Geometry check sheet. Reference: the model listing, model coordinates, mm. Face numbers are marked on the shaded views. A direction names the side the tool comes from. Round coordinates to 2 decimals unless told otherwise and drop trailing zeros. Order: outer loops, then holes, each group sorted by start corner. A loop starts at its lowest first (then second) coordinate and runs counter-clockwise, first axis right, second up.
(1) Sectioned sample at D-D (x = 63.5). Record the boundary of the cut face in (y, z), plus the area to 3 significant figures.
(2) Sectioned sample at C-C (z = -11). Record the boundary of the cut face in (x, y), plus the area to 3 significant figures.
(3) Release check for a two-part mould opening along X. For the marked faces 4, 5 and 6 record: +X half, -X half, draft (parallel to the pull), parting line (faces both ways), or undercut.
(4) Go/stop test with flat-tipped pins: pin 1 (16.5 mm diameter, centred on x = 0, y = 0, fed in from -Z); pin 2 (3 mm diameter, centred on y = -20, z = -19, fed in from +X); pin 3 (11 mm diameter, centred on x = -5.5, y = -1, fed in from -Z); pin 4 (12 mm diameter, centred on x = 68.5, z = -9, fed in from -Y). Record where each tip stops, or that it passes through.
(5) Sectioned sample at A-A (z = -32). Record the boundary of the cut face in (x, y).
(6) Sectioned sample at B-B (y = -63). Record the boundary of the cut face in (x, z), plus the area to 3 significant figures.
(7) Material ranges on line 1 along X through (y, z) = (-29, -28); line 2 along X through (y, z) = (-14, -6); line 3 along Z through (x, y) = (9, -44), recorded low to high.
(8) Set-up check for the marked faces 1, 2 and 3: record each of +Z, -Z, +X, -X, +Y, -Y from which the full face is reachable in a straight line by a thin tool's end or side.
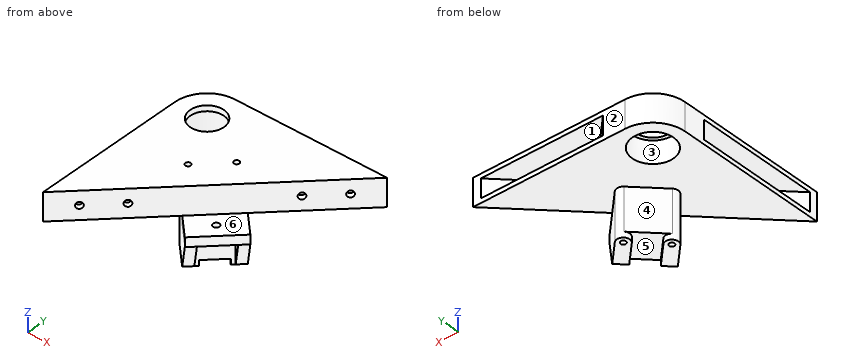
Autodesk Inventor part; units mm, degrees
ref_plane "YZ Plane" through (0, 0, 0) normal (1, 0, 0) x (0, 1, 0)
ref_plane "XZ Plane" through (0, 0, 0) normal (0, 1, 0) x (-1, 0, 0)
ref_plane "XY Plane" through (0, 0, 0) normal (0, 0, 1) x (1, 0, 0)
sketch "Sketch1" plane through (0, 0, 0) normal (0, 0, 1) x (1, 0, 0)
  circle A0 centre (0, 0) radius 4
  line L0 (-144.1925, -209.3609) -> (209.3609, 144.1925)
  circle A1 centre (0, 0) radius 11.15
  circle A2 centre (0, 0) radius 17.5
  line L1 (-17.5, 0) -> (-17.5, -82.6684)
  line L2 (0, 17.5) -> (82.6684, 17.5)
  point P0 (0, 0)
  dimension "d0" = 22.3
  dimension "d1" = 35
extrude "Extrusion1" add sketch "Sketch1" against normal blind 15 contours L1 A2 L2 L0 | A2
sketch "Sketch2" plane through (0, 0, 0) normal (0, 0, 1) x (1, 0, 0)
  arc A0 (0, 17.5) -> (-17.5, 0) centre (0, 0) ccw
  line L0 (-17.5, 0) -> (-17.5, -82.6684)
  line L1 (-17.5, -82.6684) -> (82.6684, 17.5)
  line L2 (82.6684, 17.5) -> (0, 17.5)
  circle A1 centre (0, 0) radius 11.15
  circle A2 centre (0, 0) radius 9.15
  dimension "d6" = 2
extrude "Extrusion2" add sketch "Sketch2" against normal blind 3 contours A1
ref_plane "Work Plane1" through (-19.6213, -80.5471, 0) normal (0.7071068, -0.7071068, 0) x (-0.7071068, -0.7071068, 0)
sketch "Sketch3" plane through (-19.6213, -80.5471, 0) normal (0.7071068, -0.7071068, 0) x (-0.7071068, -0.7071068, 0)
  line L0 (-141.6595, 0) -> (-83.2041, 0)
  line L1 (-141.6595, 0) -> (-141.6595, 15)
  line L2 (-83.2041, 15) -> (-141.6595, 15)
  line L3 (-83.2041, 0) -> (-83.2041, 15)
  line L4 (-58.4554, 0) -> (0, 0)
  line L5 (-58.4554, 0) -> (-58.4554, 15)
  line L6 (0, 15) -> (-58.4554, 15)
  line L7 (0, 0) -> (0, 15)
  line L8 (-83.2041, 0) -> (-58.4554, 0)
  line L9 (-50.8297, 15) -> (-90.8297, 15)
  line L10 (-141.6595, 0) -> (-141.6595, 15)
  line L11 (-141.6595, 12.6) -> (-91.6595, 12.6)
  line L12 (-91.6595, 12.6) -> (-91.6595, 2.4)
  line L13 (-91.6595, 2.4) -> (-141.6595, 2.4)
  line L14 (-141.6595, 2.4) -> (-141.6595, 12.6)
  line L15 (0, 0) -> (0, 15)
  line L16 (0, 2.4) -> (-50, 2.4)
  line L17 (-50, 2.4) -> (-50, 12.6)
  line L18 (-50, 12.6) -> (0, 12.6)
  line L19 (0, 12.6) -> (0, 2.4)
  point P0 (-70.8297, 0)
  point P1 (0, 12.6)
  dimension "d8" = 2.4
  dimension "d9" = 2.4
  dimension "d10" = 2.4
  dimension "d11" = 50
extrude "Extrusion3" cut sketch "Sketch3" against normal through all contours L1 L11 L12 L13 | L16 L17 L18 L7
sketch "Sketch4" plane through (-19.6213, -80.5471, 0) normal (-0.7071068, 0.7071068, 0) x (0, 0, 1)
  line L0 (-12.6, 138.6595) -> (-2.4, 138.6595)
  line L1 (-12.6, 91.6595) -> (-12.6, 138.6595)
  line L2 (-2.4, 91.6595) -> (-12.6, 91.6595)
  line L3 (-2.4, 138.6595) -> (-2.4, 91.6595)
  line L4 (-2.4, 3) -> (-12.6, 3)
  line L5 (-2.4, 50) -> (-2.4, 3)
  line L6 (-12.6, 50) -> (-2.4, 50)
  line L7 (-12.6, 3) -> (-12.6, 50)
  line L8 (-12.6, 50) -> (-2.4, 50)
  line L9 (-2.4, 91.6595) -> (-12.6, 91.6595)
  point P0 (0, 70.8297)
  point P1 (-7.5, 106.6595)
  point P2 (-7.5, 126.6595)
  point P3 (-7.5, 35)
  point P4 (-7.5, 15)
  point P5 (-7.5, 50)
  point P6 (-7.5, 91.6595)
  dimension "d14" = 15
  dimension "d15" = 15
  dimension "d16" = 20
  dimension "d17" = 20
hole "Hole1" at (55.7983, -5.1274, -7.5) at (69.9405, 9.0147, -7.5) at (5.1274, -55.7983, -7.5) at (-9.0147, -69.9405, -7.5) direction (0.7071068, -0.7071068, 0) diameter 3.6 end through all
sketch "Sketch5" plane through (0, 0, 0) normal (0, 0, 1) x (1, 0, 0)
  circle A0 centre (0, 0) radius 9.15
  arc A1 (0, 17.5) -> (-17.5, 0) centre (0, 0) ccw
  line L0 (-17.5, 0) -> (-17.5, -82.6684)
  line L1 (-17.5, -82.6684) -> (82.6684, 17.5)
  line L2 (82.6684, 17.5) -> (0, 17.5)
  line L3 (29, -14.8579) -> (14.8579, -29) construction
  dimension "d25" = 29
  dimension "d26" = 29
  dimension "d27" = 20
hole "Hole2" at (29, -14.8579, 0) at (14.8579, -29, 0) direction (0, 0, -1) diameter 2.9 end through all
sketch "Sketch6" plane through (0, 0, -15) normal (0, 0, -1) x (-1, 0, 0)
  circle A0 centre (-29, -14.8579) radius 1.45
  circle A1 centre (-14.8579, -29) radius 1.45
  arc A2 (17.5, 0) -> (0, 17.5) centre (0, 0) ccw
  line L0 (0, 17.5) -> (-82.6684, 17.5)
  line L1 (-82.6684, 17.5) -> (17.5, -82.6684)
  line L2 (17.5, -82.6684) -> (17.5, 0)
  circle A3 centre (0, 0) radius 11.15
  circle A4 centre (-14.8579, -29) radius 1.45
  circle A5 centre (-14.8579, -29) radius 3.5
  circle A6 centre (-29, -14.8579) radius 1.45
  circle A7 centre (-29, -14.8579) radius 3.5
  line L3 (-12.383, -31.4749) -> (-23.0382, -42.1301)
  line L4 (-17.3327, -26.5251) -> (-27.988, -37.1804)
  line L5 (-82.6684, 17.5) -> (17.5, -82.6684)
  line L6 (-31.4749, -12.383) -> (-42.1301, -23.0382)
  line L7 (-26.5251, -17.3327) -> (-37.1804, -27.988)
  point P0 (0, 0)
  dimension "d35" = 7
extrude "Extrusion4" add sketch "Sketch6" along normal blind 26 contours L1 L4 A5 L3 | L6 A7 L7 L1 | A5 | A7
sketch "Sketch7" plane through (0, 0, -15) normal (0, 0, -1) x (-1, 0, 0)
  line L0 (-26.5251, -17.3327) -> (-37.1804, -27.988)
  line L1 (-37.1804, -27.988) -> (-27.988, -37.1804)
  line L2 (-27.988, -37.1804) -> (-17.3327, -26.5251)
  arc A0 (-12.383, -31.4749) -> (-17.3327, -26.5251) centre (-14.8579, -29) ccw
  line L3 (-12.383, -31.4749) -> (-23.0382, -42.1301)
  line L4 (-23.0382, -42.1301) -> (17.5, -82.6684)
  line L5 (17.5, -82.6684) -> (17.5, 0)
  arc A1 (17.5, 0) -> (0, 17.5) centre (0, 0) ccw
  line L6 (0, 17.5) -> (-82.6684, 17.5)
  line L7 (-82.6684, 17.5) -> (-42.1301, -23.0382)
  line L8 (-42.1301, -23.0382) -> (-31.4749, -12.383)
  arc A2 (-26.5251, -17.3327) -> (-31.4749, -12.383) centre (-29, -14.8579) ccw
  circle A3 centre (0, 0) radius 11.15
  line L9 (-12.383, -26.5251) -> (-26.5251, -12.383)
  arc A4 (-26.5251, -17.3327) -> (-31.4749, -12.383) centre (-29, -14.8579) ccw
  point P0 (0, 0)
extrude "Extrusion5" add sketch "Sketch7" along normal blind 23 contours A2 L9 A0 L2 L1 L0
sketch "Sketch8" plane through (-17.5, -82.6684, 0) normal (0.7071068, -0.7071068, 0) x (-0.7071068, -0.7071068, 0)
  circle A0 centre (-35, 7.5) radius 1.8
  circle A1 centre (-106.6595, 7.5) radius 1.8
  circle A2 centre (-126.6595, 7.5) radius 1.8
  circle A3 centre (-15, 7.5) radius 1.8
  line L0 (0, 0) -> (-141.6595, 0)
  line L1 (0, 0) -> (0, 15)
  line L2 (-57.3297, 15) -> (0, 15)
  line L3 (-57.3297, 15) -> (-57.3297, 41)
  line L4 (-64.3297, 41) -> (-57.3297, 41)
  line L5 (-64.3297, 38) -> (-64.3297, 41)
  line L6 (-77.3297, 38) -> (-64.3297, 38)
  line L7 (-77.3297, 38) -> (-77.3297, 41)
  line L8 (-84.3297, 41) -> (-77.3297, 41)
  line L9 (-84.3297, 15) -> (-84.3297, 41)
  line L10 (-141.6595, 15) -> (-84.3297, 15)
  line L11 (-141.6595, 0) -> (-141.6595, 15)
  line L12 (-84.3297, 15) -> (-57.3297, 15)
  line L13 (-83.2041, 15) -> (-141.6595, 15)
  line L14 (-84.3297, 15) -> (-84.3297, 41)
  line L15 (-84.3297, 20) -> (-57.3297, 20)
  point P0 (-70.8297, 0)
  dimension "d40" = 5
extrude "Extrusion6" add sketch "Sketch8" along normal blind 15 contours L12 L9 L15 L3
sketch "Sketch9" plane through (31.4749, -12.383, -41) normal (0.7071068, 0.7071068, 0) x (-0.7071068, 0.7071068, 0)
  line L0 (-15.0688, 26) -> (0, 26)
  line L1 (-15.0688, 26) -> (-30.0688, 26)
  line L2 (-30.0688, 21) -> (-30.0688, 26)
  line L3 (-15.0688, 21) -> (-30.0688, 21)
  line L4 (-15.0688, 21) -> (-15.0688, 0)
  line L5 (0, 0) -> (-15.0688, 0)
  line L6 (0, 26) -> (0, 0)
  line L7 (-15.0688, 0) -> (-30.0688, 21)
  point P0 (31.0122, 41)
extrude "Extrusion7" add sketch "Sketch9" against normal blind 5 contours L3 L4 L7
sketch "Sketch10" plane through (12.383, -31.4749, -15) normal (-0.7071068, -0.7071068, 0) x (-0.7071068, 0.7071068, 0)
  line L0 (-15.0688, 26) -> (-30.0688, 5)
  line L1 (-15.0688, 5) -> (-30.0688, 5)
  line L2 (-15.0688, 26) -> (-15.0688, 5)
  point P0 (31.0122, -15)
extrude "Extrusion8" add sketch "Sketch10" against normal blind 5
sketch "Sketch11" plane through (49.2012, -37.1804, -20) normal (0, 0, -1) x (-0.7071068, -0.7071068, 0)
  line L0 (17, 0) -> (17, 15)
  line L1 (0, 15) -> (17, 15)
  line L2 (0, 15) -> (0, 0)
  line L3 (17, 0) -> (0, 0)
  line L4 (2, 15) -> (15, 15)
  point P0 (8.5, 61.081)
  point P1 (8.5, 7.5)
  point P2 (0, 7.5)
  point P3 (8.5, 15)
hole "Hole3" at (37.8875, -37.8875, -20) direction (0, 0, 1) diameter 3.5 end through all
equation "\"d9\" = d8"
equation "\"d10\" = d8"
properties part number "Rear Z Axis Bottom Bearing" material "ABS Plastic"
Answer below:
1. outline: (-1.67, -15) - (17.5, -15) - (17.5, -12.6) - (2.57, -12.6) - (2.57, -2.4) - (17.5, -2.4) - (17.5, 0) - (-1.67, 0) - close
1. area: 135 mm2
2. outline: (-17.5, -82.67) - (82.67, 17.5) - (78.43, 17.5) - (45.19, -15.73) - (11.96, 17.5) - (0, 17.5) arc R17.5 ccw to (-17.5, 0) - (-17.5, -11.96) - (15.73, -45.19) - (-17.5, -78.43) - close; hole circle Ø22.3 at (0, 0); hole circle Ø2.9 at (14.86, -29); hole circle Ø2.9 at (29, -14.86)
2. area: 2,340 mm2
3. face 4: -X half
3. face 5: undercut
3. face 6: draft
4. pin 1: passes through
4. pin 2: stops at x = 40.59
4. pin 3: stops at z = -3
4. pin 4: stops at y = -2.67
5. outline: (12.38, -31.47) - (27.58, -46.68) - (31.12, -43.14) - (26.57, -38.59) - (38.59, -26.57) - (43.14, -31.12) - (46.68, -27.58) - (31.47, -12.38) arc R3.5 ccw to (26.53, -12.38) - (12.38, -26.53) arc R3.5 ccw to start; hole circle Ø2.9 at (14.86, -29); hole circle Ø2.9 at (29, -14.86)
6. outline: (-17.5, -15) - (2.17, -15) - (2.17, 0) - (-17.5, 0) - (-17.5, -2.4) - (-2.07, -2.4) - (-2.07, -12.6) - (-17.5, -12.6) - close
6. area: 138 mm2
7. line 1: x = 11.36 to 13.41, 16.31 to 36.17, 41.02 to 48.09
7. line 2: x = -15.46 to 27.83, 30.17 to 43.46, 46.93 to 51.17
7. line 3: z = -15 to -12.6, -2.4 to 0
8. face 1: +Y
8. face 2: +Z, -Z, +X, -X, +Y
8. face 3: -Z
